Verification items for the finished model (mm, model axes). A direction names the side the tool comes from. Give positions to 0.01 mm unless a question says otherwise; leave off trailing zeros. Write each loop counter-clockwise with the first axis right and the second up, starting at its lowest first coordinate (ties: lowest second). Pieces come first, ordered by that corner, then holes. Notation, with made-up numbers: M 3,43.25 L 25,43.25 A21 ccw 25,68.25 Z; hole C 73,25 d5. An arc over 180 degrees is marked long. Answer as a JSON object with one key per item and string values.
```python
from build123d import *

# Parameters (mm, degrees)
SKETCH1_W           = 50
SKETCH1_H           = 42
BOSS_EXTRUDE1_DEPTH = 40
FILLET1_R           = 21
FILLET2_R           = 16
BOSS_EXTRUDE2_REACH = 96.81
SKETCH2_R           = 20
CHAMFER1_SIZE       = 2.5
SKETCH3_R           = 5
CUT_EXTRUDE1_DEPTH  = 10
SKETCH4_R           = 5
BOSS_EXTRUDE3_DEPTH = 10


with BuildPart() as part:
    # Sketch1 → Boss-Extrude1 (new body)
    with BuildSketch(Plane(origin=(0, 0, 0), x_dir=(1, 0, 0), z_dir=(0, 1, 0))):
        with Locations((25, 21)):
            Rectangle(SKETCH1_W, SKETCH1_H)
    extrude(amount=BOSS_EXTRUDE1_DEPTH)

    # Fillet1
    # the kernel refuses this fillet: 21 mm, written as the material it takes off along each edge
    with BuildSketch(Plane(origin=(0, 0, -94.5), x_dir=(0, 1, 0), z_dir=(0, 0, 1))) as fillet1_piece_1:
        with BuildLine():
            CenterArc((FILLET1_R, -FILLET1_R), FILLET1_R, 90, 90)
            Line((0, -FILLET1_R), (0, 0))
            Line((0, 0), (FILLET1_R, 0))
        make_face()
    extrude(amount=147, mode=Mode.SUBTRACT)
    with BuildSketch(Plane(origin=(0, 40, -94.5), x_dir=(0, -1, 0), z_dir=(0, 0, 1))) as fillet1_piece_2:
        with BuildLine():
            CenterArc((FILLET1_R, FILLET1_R), FILLET1_R, 180, 90)
            Line((0, FILLET1_R), (0, 0))
            Line((0, 0), (FILLET1_R, 0))
        make_face()
    extrude(amount=147, mode=Mode.SUBTRACT)

    # Fillet2
    fillet2_edges = [part.edges().sort_by_distance(p)[0] for p in [
        (50, 40, -21),
        (50, 0, -21),
    ]]
    fillet(fillet2_edges, radius=FILLET2_R)

    # Sketch2 → Boss-Extrude2 (add, up to next)
    with BuildSketch(Plane.ZY.offset(25), mode=Mode.PRIVATE) as boss_extrude2_sk1:
        with Locations((-21, 20)):
            Circle(SKETCH2_R)
    boss_extrude2_tool1 = extrude(boss_extrude2_sk1.sketch, amount=-BOSS_EXTRUDE2_REACH, mode=Mode.PRIVATE) - part.part
    add(boss_extrude2_tool1.solids().sort_by_distance((-25, 20, -21))[0])

    # Chamfer1
    # the kernel refuses this chamfer: 2.5 mm, written as the material it takes off along each edge
    with BuildSketch(Plane(origin=(21, 40, 0), x_dir=(0, -0.9996219169112968, 0.027495876610586334), z_dir=(1, 0, 0)), Plane(origin=(34, 0, -42), x_dir=(0, -0.027495876610586334, 0.9996219169112968), z_dir=(-1, 0, 0))) as chamfer1_piece_1:
        Polygon((CHAMFER1_SIZE * 0.999621916911, CHAMFER1_SIZE * 0.0274958766106), (-CHAMFER1_SIZE * 0.0274958766106, CHAMFER1_SIZE * 0.999621916911), (0, 0), align=None)
    extrude(amount=13, mode=Mode.SUBTRACT)
    with BuildSketch(Plane(origin=(34, 24, 0), x_dir=(1, 0, 0), z_dir=(0, -1, 0))) as chamfer1_piece_2:
        Polygon((16 - CHAMFER1_SIZE, 0), (16, -CHAMFER1_SIZE), (16, 0), align=None)
    revolve(axis=Axis((34, 24, 0), (0, 0, 1)), revolution_arc=90, mode=Mode.SUBTRACT)
    with BuildSketch(Plane(origin=(21, 19, 0), x_dir=(-0.9667409364669165, -0.25575762307127703, 0), z_dir=(0.25575762307127703, -0.9667409364669165, 0))) as chamfer1_piece_3_section:
        Polygon((21 - CHAMFER1_SIZE, 0), (21, CHAMFER1_SIZE), (21, 0), align=None)
    chamfer1_piece_3 = revolve(axis=Axis((21, 19, 0), (0, 0, -1)), revolution_arc=104.818482505, mode=Mode.PRIVATE)
    chamfer1_piece_3 = chamfer1_piece_3 - Plane(origin=(5.32298007, 20, -21), x_dir=(0, 0, 1), z_dir=(-1, 0, 0)) * Cylinder(20, 85, mode=Mode.PRIVATE)
    add(chamfer1_piece_3, mode=Mode.SUBTRACT)
    with BuildSketch(Plane(origin=(50, 16, 0), x_dir=(-0.9996219169112968, 0, 0.027495876610586334), z_dir=(0, 1, 0)), Plane(origin=(50, 16, -42), x_dir=(0.027495876610587663, 0, 0.9996219169112968), z_dir=(0, 1, 0))) as chamfer1_piece_4:
        Polygon((CHAMFER1_SIZE * 0.999621916911, -CHAMFER1_SIZE * 0.0274958766106), (-CHAMFER1_SIZE * 0.0274958766106, -CHAMFER1_SIZE * 0.999621916911), (0, 0), align=None)
    extrude(amount=8, mode=Mode.SUBTRACT)
    with BuildSketch(Plane(origin=(21, 21, 0), x_dir=(0, -1, 0), z_dir=(1, 0, 0))) as chamfer1_piece_5_section:
        Polygon((21 - CHAMFER1_SIZE, 0), (21, CHAMFER1_SIZE), (21, 0), align=None)
    chamfer1_piece_5 = revolve(axis=Axis((21, 21, 0), (0, 0, -1)), revolution_arc=104.818482505, mode=Mode.PRIVATE)
    chamfer1_piece_5 = chamfer1_piece_5 - Plane(origin=(5.322980064, 20, -21), x_dir=(0, 0, 1), z_dir=(-1, 0, 0)) * Cylinder(20, 84, mode=Mode.PRIVATE)
    add(chamfer1_piece_5, mode=Mode.SUBTRACT)
    with BuildSketch(Plane(origin=(34, 16, 0), x_dir=(0, -1, 0), z_dir=(-1, 0, 0))) as chamfer1_piece_6:
        Polygon((16 - CHAMFER1_SIZE, 0), (16, -CHAMFER1_SIZE), (16, 0), align=None)
    revolve(axis=Axis((34, 16, 0), (0, 0, 1)), revolution_arc=90, mode=Mode.SUBTRACT)
    with BuildSketch(Plane(origin=(21, 0, 0), x_dir=(0, 0.9996219169112968, 0.027495876610586372), z_dir=(1, 0, 0)), Plane(origin=(34, 40, -42), x_dir=(0, 0.027495876610587663, 0.9996219169112968), z_dir=(-1, 0, 0))) as chamfer1_piece_7:
        Polygon((CHAMFER1_SIZE * 0.999621916911, -CHAMFER1_SIZE * 0.0274958766106), (-CHAMFER1_SIZE * 0.0274958766106, -CHAMFER1_SIZE * 0.999621916911), (0, 0), align=None)
    extrude(amount=13, mode=Mode.SUBTRACT)
    with BuildSketch(Plane(origin=(34, 24, -42), x_dir=(1, 0, 0), z_dir=(0, -1, 0))) as chamfer1_piece_8:
        Polygon((16, CHAMFER1_SIZE), (16 - CHAMFER1_SIZE, 0), (16, 0), align=None)
    revolve(axis=Axis((34, 24, -42), (0, 0, 1)), revolution_arc=90, mode=Mode.SUBTRACT)
    with BuildSketch(Plane(origin=(21, 19, -42), x_dir=(-0.9667409364669164, -0.25575762307127753, 0), z_dir=(0.25575762307127753, -0.9667409364669164, 0))) as chamfer1_piece_9_section:
        Polygon((21 - CHAMFER1_SIZE, 0), (21, -CHAMFER1_SIZE), (21, 0), align=None)
    chamfer1_piece_9 = revolve(axis=Axis((21, 19, -42), (0, 0, -1)), revolution_arc=104.818482505, mode=Mode.PRIVATE)
    chamfer1_piece_9 = chamfer1_piece_9 - Plane(origin=(5.322980068, 20, -21), x_dir=(0, 0, 1), z_dir=(-1, 0, 0)) * Cylinder(20, 85, mode=Mode.PRIVATE)
    add(chamfer1_piece_9, mode=Mode.SUBTRACT)
    with BuildSketch(Plane(origin=(34, 16, -42), x_dir=(0, -1, 0), z_dir=(-1, 0, 0))) as chamfer1_piece_10:
        Polygon((16, CHAMFER1_SIZE), (16 - CHAMFER1_SIZE, 0), (16, 0), align=None)
    revolve(axis=Axis((34, 16, -42), (0, 0, 1)), revolution_arc=90, mode=Mode.SUBTRACT)
    with BuildSketch(Plane(origin=(21, 21, -42), x_dir=(0, -1, 0), z_dir=(1, 0, 0))) as chamfer1_piece_11_section:
        Polygon((21 - CHAMFER1_SIZE, 0), (21, -CHAMFER1_SIZE), (21, 0), align=None)
    chamfer1_piece_11 = revolve(axis=Axis((21, 21, -42), (0, 0, -1)), revolution_arc=104.818482505, mode=Mode.PRIVATE)
    chamfer1_piece_11 = chamfer1_piece_11 - Plane(origin=(5.322980065, 20, -21), x_dir=(0, 0, 1), z_dir=(-1, 0, 0)) * Cylinder(20, 84, mode=Mode.PRIVATE)
    add(chamfer1_piece_11, mode=Mode.SUBTRACT)

    # Sketch3 → Cut-Extrude1 (cut)
    with BuildSketch(Plane.XY):
        with Locations((21.525657906, 20)):
            Circle(SKETCH3_R)
    extrude(amount=-CUT_EXTRUDE1_DEPTH, mode=Mode.SUBTRACT)

    # Sketch4 → Boss-Extrude3 (add)
    with BuildSketch(Plane.ZY.offset(25)):
        with Locations((-21, 20)):
            Circle(SKETCH4_R)
    extrude(amount=BOSS_EXTRUDE3_DEPTH)


solid = part.part
```
1) Access from +Z, -Z, +X, -X, +Y, -Y to the whole of each face (thin tool, end or side, straight path). Record for faces 5 (the face through (14.6, 39, -34.5)), 6 (the face through (14.251, 1.114, -34.491)), 7 (the face through (27, 0, -21)), 8 (the face through (14.251, 1.114, -7.768)).
Completed:
{"face 5": "-Z, -X, +Y", "face 6": "-Z, -X, -Y", "face 7": "+Z, -Z, +X, -X, -Y", "face 8": "+Z, -X, -Y"}
2) Go/stop test with flat-tipped pins: pin 1 (1 mm diameter, centred on x = -20, z = -25, fed in from -Y); pin 2 (5 mm diameter, centred on x = 21.5, y = 21.5, fed in from +Z); pin 3 (4 mm diameter, centred on x = 6.5, y = 4.5, fed in from -Z). Record where each tip stops, or that it passes through.
Completed:
{"pin 1": "stops at y = 0.31", "pin 2": "stops at z = -10", "pin 3": "stops at z = -40.53"}
3) Thickness scan on L1, parallel to Z at x = 1, y = 19.5; L2, parallel to Y at x = 17, z = -9; L3, parallel to Y at x = -24.5, z = -21. Record the ranges inside material, lowest first.
Completed:
{"L1": "z = -40.99 to -1.01", "L2": "y = 0.38 to 17.87, 22.13 to 39.62", "L3": "y = 0 to 40"}
4) Section check B-B on z = -24.5. Record the boundary of the cut face in (x, y), and give its area (3 significant figures).
Completed:
{"outline": "M -35,16.43 L -25,16.43 L -25,0.31 L 17.41,0.31 A21 ccw 21,0 L 34,0 A16 ccw 50,16 L 50,24 A16 ccw 34,40 L 21,40 A21 ccw 17.41,39.69 L -25,39.69 L -25,23.57 L -35,23.57 Z", "area": "2,930 mm2"}
5) Section check A-A on z = -9. Record the boundary of the cut face in (x, y), and give its area (3 significant figures).
Completed:
{"outline": "M -25,4 L 8.67,4 A21 ccw 21,0 L 34,0 A16 ccw 50,16 L 50,24 A16 ccw 34,40 L 21,40 A21 ccw 8.67,36 L -25,36 Z; hole C 21.53,20 d10", "area": "2,510 mm2"}
6) Release check for a two-part mould opening along X. For faces 1 (the face through (21, 20, -10)), 2 (the face through (23.833, 15.564, -4.93)), 3 (the face through (8.106, 7.135, -41.566)), 4 (the face through (43.94, 33.72, -41.6)) record: pulls with the +X half, pulls with the -X half, needs draft (parallel to the pull), parting line crosses it, or undercut.
Completed:
{"face 1": "undercut", "face 2": "undercut", "face 3": "pulls with the -X half", "face 4": "pulls with the +X half"}
7) Section check C-C on z = -15. Record the boundary of the cut face in (x, y).
Completed:
{"outline": "M -25,0.92 L 14.85,0.92 A21 ccw 21,0 L 34,0 A16 ccw 50,16 L 50,24 A16 ccw 34,40 L 21,40 A21 ccw 14.85,39.08 L -25,39.08 Z"}
